Part print with two shaded views. Sizes in mm from the minimum x, y, z corner. A direction names the side the tool comes from. Coordinates: 2 decimals unless noted, no trailing zeros. Write each loop counter-clockwise with the first axis right and the second up, starting at its lowest first coordinate (ties: lowest second). Pieces come first, ordered by that corner, then holes. Notation, with made-up numbers: (69.25, 10) - (123.25, 10) arc R21 cw to (123.25, 27) - close; hole circle Ø5 at (7, -2). An arc over 180 degrees is marked (long way). One line per question, with ' | ' between items. Start each with the question number.
1. Band-saw the part on B-B, the plane x = 8.5. Write the cut outline in (y, z), then the cut area to 3 significant figures.
2. Which spindle directions (+Z, -Z, +X, -X, +Y, -Y) get a long thin tool onto all of the face, cutting with end or side? Do the marked faces 1, 2, 3 and 4. Say none if no direction does.
3. Probe line 1 (Y direction, x = 10, z = 2.75); line 2 (X direction, y = 15, z = 9.25); line 3 (X direction, y = 2.5, z = 2.75). List the from-to ranges inside material, lowest first.
4. Band-saw the part on D-D, the plane x = 4. Write the cut outline in (y, z).
5. Band-saw the part on C-C, the plane z = 4.75. Write the cut outline in (x, y), then the cut area to 3 significant figures.
6. Two-plate mould, pull along Y, no slides. Class the marked faces 5, 6 and 7: +Y half, -Y half, draft (parallel to the pull), parting line (faces both ways), or undercut.
7. Flat gauge pins, fed straight in: P1, Ø4.5, axis at x = 11.5, z = 4.5, coming from the -Y side; P2, Ø2, axis at x = 5.5, z = 3, coming from the -Y side. Where does each tip first touch, or does it go through?
8. Band-saw the part on A-A, the plane y = 18.5. Write the cut outline in (x, z), then the cut area to 3 significant figures.
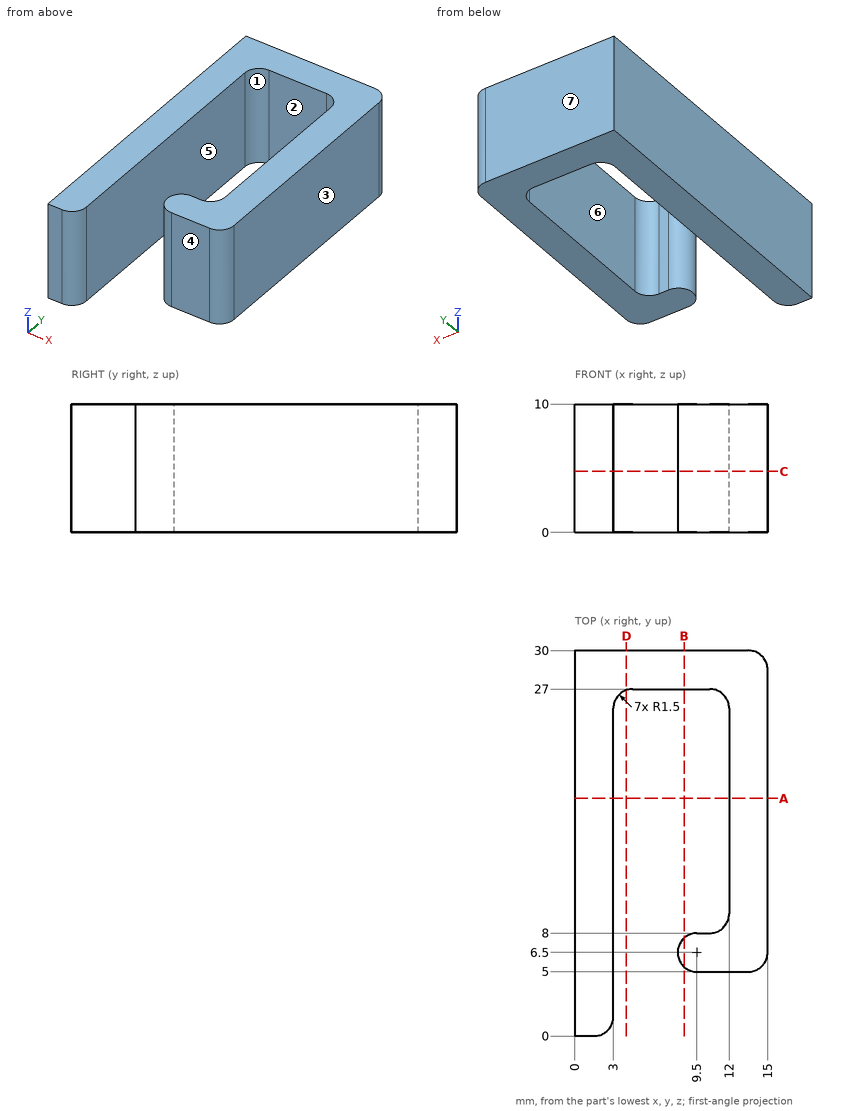
Filled in:
1) outline: (5.38, 0) - (7.62, 0) - (7.62, 10) - (5.38, 10) - close; (27, 0) - (30, 0) - (30, 10) - (27, 10) - close | area: 52.4 mm²
2) face 1: +Z, -Z, -Y | face 2: +Z, -Z | face 3: +Z, -Z, +X, +Y, -Y | face 4: +Z, -Z, +X, -Y
3) line 1: y = 5 to 8, 27 to 30 | line 2: x = 0 to 3, 12 to 15 | line 3: x = 0 to 3
4) outline: (26.91, 0) - (30, 0) - (30, 10) - (26.91, 10) - close
5) outline: (0, 0) - (1.5, 0) arc R1.5 ccw to (3, 1.5) - (3, 25.5) arc R1.5 cw to (4.5, 27) - (10.5, 27) arc R1.5 cw to (12, 25.5) - (12, 9.5) arc R1.5 cw to (10.5, 8) - (9.5, 8) arc R1.5 ccw to (9.5, 5) - (13.5, 5) arc R1.5 ccw to (15, 6.5) - (15, 28.5) arc R1.5 ccw to (13.5, 30) - (0, 30) - close | area: 203 mm²
6) face 5: draft | face 6: undercut | face 7: +Y half
7) P1: stops at y = 5 | P2: stops at y = 27
8) outline: (0, 0) - (3, 0) - (3, 10) - (0, 10) - close; (12, 0) - (15, 0) - (15, 10) - (12, 10) - close | area: 60.0 mm²
